```python
from build123d import *

# Parameters (mm, degrees)
SKETCH_R        = 3.4
SKETCH_R_2      = 1.9
PAD_DEPTH       = 10
CHAMFER_SIZE2   = 1
CHAMFER_SIZE    = 6
PAD001_START    = -2.6
SKETCH001_R     = 3.65
SKETCH001_R_2   = 3.4
PAD001_DEPTH    = 1.4
SKETCH002_R     = 3.65
SKETCH002_R_2   = 3.4
PAD002_DEPTH    = 0.5
CHAMFER001_SIZE = 0.24


with BuildPart() as part:
    # Sketch → Pad (new body)
    with BuildSketch(Plane.XY):
        Circle(SKETCH_R)
        Circle(SKETCH_R_2, mode=Mode.SUBTRACT)
    extrude(amount=PAD_DEPTH)

    # Chamfer
    chamfer_edges = [part.edges().sort_by_distance(p)[0] for p in [
        (-3.4, 0, 10),
    ]]
    chamfer_side = part.faces().sort_by_distance((-3.4, 0, 5))[0]
    chamfer(chamfer_edges, length=CHAMFER_SIZE, length2=CHAMFER_SIZE2, reference=chamfer_side)

    # Sketch001 (on Face3 of Chamfer) → Pad001 (join)
    with BuildSketch(Plane(origin=(0, 0, 0), x_dir=(1, 0, 0), z_dir=(0, 0, -1)).offset(PAD001_START)):
        Circle(SKETCH001_R)
        Circle(SKETCH001_R_2, mode=Mode.SUBTRACT)
    extrude(amount=-PAD001_DEPTH)

    # Sketch002 (on Face2 of Pad001) → Pad002 (join)
    with BuildSketch(Plane(origin=(0, 0, 0), x_dir=(1, 0, 0), z_dir=(0, 0, -1))):
        Circle(SKETCH002_R)
        Circle(SKETCH002_R_2, mode=Mode.SUBTRACT)
    extrude(amount=-PAD002_DEPTH)

    # Chamfer001
    chamfer001_edges = [part.edges().sort_by_distance(p)[0] for p in [
        (-3.65, 0, 4),
    ]]
    chamfer(chamfer001_edges, length=CHAMFER001_SIZE)


solid = part.part
```
The listing builds one solid part. Answer for the finished solid, in the listing's coordinates (mm). Give positions to 0.01 mm unless a question says otherwise; leave off trailing zeros. Order: outer loops, then holes, each group sorted by start corner. A loop starts at its lowest first (then second) coordinate and runs counter-clockwise, first axis right, second up. Notation, with made-up numbers: (10.5, -37.75) -> (41.5, -37.75) arc R27 cw to (41.5, -7.75) -> close; hole circle Ø8 at (81, 75.5). An arc over 180 degrees is marked (long way). One line per item, written item: value.
1) Flat-ended cylindrical pins translate along their axes: P1, Ø1.5, axis at y = 2, z = 8.5, coming from the -X side; P2, Ø1.5, axis at x = -2, z = 4, coming from the -Y side; P3, Ø3, axis at x = 0, y = 0, coming from the -Z side; P4, Ø4, axis at y = 0, z = 2, coming from the -X side. Find the tip coordinate at first contact, or state that the pin passes through.
Reported:
P1: stops at x = -2.36
P2: stops at y = -3.41
P3: passes through
P4: stops at x = -3.65
2) Find section C-C, the plane z = 2. Determine the outline of the cut face in (x, y).
Reported:
outline: circle Ø6.8 at (0, 0); hole circle Ø3.8 at (0, 0)
3) Determine the mould class of faces 1 (the cylindrical face through (3.48, -1.1, 3.17)), 2 (the cylindrical face through (-0.74, -3.32, 1.54)), 3 (the flat face through (2, 1, 10)) for opening direction Z: pulls with the +Z half, pulls with the -Z half, needs draft (parallel to the pull), parting line crosses it, or undercut.
Reported:
face 1: needs draft
face 2: undercut
face 3: pulls with the +Z half
4) Find section D-D, the plane z = 3.25. Determine the outline of the cut face in (x, y), plus the area to 3 significant figures.
Reported:
outline: circle Ø7.3 at (0, 0); hole circle Ø3.8 at (0, 0)
area: 30.5 mm^2
5) Find the intervals of material crossed by line 1 (Y direction, x = 0, z = 3); line 2 (Y direction, x = 0, z = 2.5); line 3 (X direction, y = 1.25, z = 7.25), in increasing order.
Reported:
line 1: y = -3.65 to -1.9, 1.9 to 3.65
line 2: y = -3.4 to -1.9, 1.9 to 3.4
line 3: x = -2.57 to -1.43, 1.43 to 2.57
